Solid Edge part; units mm, degrees
sketch "Sketch1" plane through (0, 0, 0) normal (0, -1, 0) x (1, 0, 0)
  line L0 (21.3868, 29.4641) -> (-66.4383, 29.4641)
  arc A0 (-110, -14.0976) -> (-66.4383, 29.4641) centre (-66.4383, -14.0976) cw
  line L1 (-110, -14.0976) -> (-110, -100.5359)
  line L2 (-110, -100.5359) -> (110, -100.5359)
  line L3 (110, -100.5359) -> (110, -59.1492)
  arc A1 (21.3868, 29.4641) -> (110, -59.1492) centre (21.3868, -59.1492) cw
  line L4 (-78.3036, 12.5363) -> (-58.5498, 15.665)
  line L5 (-58.5498, 15.665) -> (-57.9241, 11.7142)
  line L6 (-57.9241, 11.7142) -> (-77.6778, 8.5855)
  line L7 (-77.6778, 8.5855) -> (-78.3036, 12.5363)
  line L8 (-38.796, 18.7936) -> (-19.0423, 21.9223)
  line L9 (-19.0423, 21.9223) -> (-18.4165, 17.9716)
  line L10 (-18.4165, 17.9716) -> (-38.1703, 14.8429)
  line L11 (-38.1703, 14.8429) -> (-38.796, 18.7936)
  line L12 (-98.4684, -0.7822) -> (-93.5299, 0)
  line L13 (-93.5299, 0) -> (-90.4012, -19.7538)
  line L14 (-90.4012, -19.7538) -> (-95.3397, -20.5359)
  line L15 (-95.3397, -20.5359) -> (-98.4684, -0.7822)
extrude "Protrusion1" add sketch "Sketch1" against normal blind 4
The listing builds one solid part. Answer for the finished solid, in the listing's coordinates (mm). A direction names the side the tool comes from. Coordinates: 2 decimals unless noted, no trailing zeros. Write each loop counter-clockwise with the first axis right and the second up, starting at its lowest first coordinate (ties: lowest second). Pieces come first, ordered by that corner, then holes. Notation, with made-up numbers: (69.5, -32.75) - (99.5, -32.75) arc R10 ccw to (99.5, -16.75) - close; hole circle Ø10 at (77, 8.5). An arc over 180 degrees is marked (long way). Return JSON: item names as keys, results as strings.
1. Which of the six approach directions +Z, -Z, +X, -X, +Y, -Y give full straight-line access (tool end or side, diameter ignored) to faces 1 (the face through (-58.24, 1.97, 13.72)), 2 (the face through (-96.9, 1.97, 17.04))?
Final values:
{"face 1": "+Y, -Y", "face 2": "+Z, -X, +Y, -Y"}
2. Each of these flat-tipped pins is pushed along its axis until it touches: pin 1 Ø2 at (y, z) = (1.5, 12) entering from +X; pin 2 Ø2 at (x, z) = (-9, -9.5) entering from -Y. Where does it stop, or does it pass through?
Final values:
{"pin 1": "x = 75.53", "pin 2": "y = 0"}
3. The part is cut by section B-B on x = -30.5. Determine the outline of the cut face in (y, z), then the cut area to 3 significant figures.
Final values:
{"outline": "(0, -100.54) - (4, -100.54) - (4, 16.06) - (0, 16.06) - close; (0, 20.11) - (4, 20.11) - (4, 29.46) - (0, 29.46) - close", "area": "504 mm^2"}
4. Consider line 1 along X through (y, z) = (0.4, -6.5); line 2 along X through (y, z) = (0.65, -35.5); line 3 along X through (y, z) = (1.4, 12). Determine where each line is inside the solid, lowest interval first.
Final values:
{"line 1": "-109.33 to -97.56, -92.5 to 92.66", "line 2": "-110 to 106.79", "line 3": "-101.32 to -78.22, -57.97 to 74.21"}
5. The part is cut by section A-A on y = 2. Determine the outline of the cut face in (x, z) (1 decimal).
Final values:
{"outline": "(-110, -100.5) - (110, -100.5) - (110, -59.1) arc R88.6 ccw to (21.4, 29.5) - (-66.4, 29.5) arc R43.6 ccw to (-110, -14.1) - close; hole (-98.5, -0.8) - (-95.3, -20.5) - (-90.4, -19.8) - (-93.5, 0) - close; hole (-78.3, 12.5) - (-77.7, 8.6) - (-57.9, 11.7) - (-58.5, 15.7) - close; hole (-38.8, 18.8) - (-38.2, 14.8) - (-18.4, 18) - (-19, 21.9) - close"}
6. The part is cut by section C-C on x = -84. Determine the outline of the cut face in (y, z), then the cut area to 3 significant figures.
Final values:
{"outline": "(0, -100.54) - (4, -100.54) - (4, 25.77) - (0, 25.77) - close", "area": "505 mm^2"}
7. The part is cut by section D-D on x = 50. Determine the outline of the cut face in (y, z), then the cut area to 3 significant figures.
Final values:
{"outline": "(0, -100.54) - (4, -100.54) - (4, 24.72) - (0, 24.72) - close", "area": "501 mm^2"}
